Autodesk Inventor part; units mm, degrees
ref_plane "YZ Plane" through (0, 0, 0) normal (1, 0, 0) x (0, 1, 0)
ref_plane "XZ Plane" through (0, 0, 0) normal (0, 1, 0) x (-1, 0, 0)
ref_plane "XY Plane" through (0, 0, 0) normal (0, 0, 1) x (1, 0, 0)
sketch "Szkic1" plane through (0, 0, 0) normal (0, 1, 0) x (-1, 0, 0)
  line L0 (0, 0) -> (0, -35)
  circle A0 centre (0, 0) radius 2
  circle A1 centre (0, -35) radius 2
  line L1 (0, 0) -> (0, -35) construction
  line L2 (-25, 0) -> (-25, -35)
  line L3 (25, -35) -> (25, 0)
  arc A2 (25, 0) -> (-25, 0) centre (0, 0) ccw
  arc A3 (-25, -35) -> (25, -35) centre (0, -35) ccw
  line L4 (-20, -45) -> (20, -45)
  line L5 (20, -45) -> (20, -25)
  line L6 (20, -25) -> (-20, -25)
  line L7 (-20, -25) -> (-20, -45)
  line L8 (-20, -45) -> (20, -25) construction
  line L9 (20, -45) -> (-20, -25) construction
  line L10 (0, -17.5) -> (-25, -17.5) construction
  line L11 (0, -35) -> (0, 0)
  circle A4 centre (0, 0) radius 2
  line L12 (0, -35) -> (0, 0) construction
  line L13 (-20, 10) -> (20, 10)
  line L14 (20, 10) -> (20, -10)
  line L15 (20, -10) -> (-20, -10)
  line L16 (-20, 10) -> (20, -10) construction
  line L17 (20, 10) -> (-20, -10) construction
  line L18 (-20, -10) -> (-20, 10)
  line L19 (0, -17.5) -> (-400, -17.5) construction
  line L20 (0, -17.5) -> (400, -17.5) construction
  line L21 (21.5, 12.5) -> (-21.5, 12.5)
  line L22 (-21.5, 12.5) -> (-21.5, -47.5)
  line L23 (-21.5, -47.5) -> (21.5, -47.5)
  line L24 (21.5, -47.5) -> (21.5, 12.5)
  line L25 (21.5, 12.5) -> (-21.5, -47.5) construction
  line L26 (-21.5, 12.5) -> (21.5, -47.5) construction
  line L27 (21.5, -47.5) -> (28.5, -47.5)
  line L28 (28.5, -47.5) -> (28.5, 12.5)
  line L29 (28.5, 12.5) -> (21.5, 12.5)
  line L30 (21.5, 12.5) -> (21.5, -47.5)
  line L31 (20, 10) -> (20, -10)
  line L32 (20, 0) -> (20, -10)
  circle A5 centre (25, -5) radius 2
  line L33 (20, 0) -> (28.5, 0) construction
  circle A6 centre (25, 5) radius 2
  circle A7 centre (-25, -5) radius 2
  circle A8 centre (-25, 5) radius 2
  line L34 (-21.5, -47.5) -> (-21.5, 12.5)
  line L35 (-21.5, -47.5) -> (-28.5, -47.5)
  line L36 (-28.5, -47.5) -> (-28.5, 12.5)
  line L37 (-28.5, 12.5) -> (-21.5, 12.5)
  circle A9 centre (25, -30) radius 2
  circle A10 centre (25, -40) radius 2
  circle A11 centre (-25, -30) radius 2
  circle A12 centre (-25, -40) radius 2
  point P0 (20, -5)
  dimension "d0" = 35
  dimension "d1" = 4
  dimension "d2" = 4
  dimension "d3" = 50
  dimension "d6" = 40
  dimension "d7" = 20
  dimension "d8" = 400
  dimension "d9" = 180
  dimension "d10" = 43
  dimension "d11" = 60
  dimension "d21" = 7
  dimension "d22" = 60
  dimension "d24" = 4
  dimension "d25" = 5
  dimension "d26" = 5
extrude "Wyciągnięcie proste1" add sketch "Szkic1" against normal blind 5 contours L21 L24 L23 L22
sketch "Szkic2" plane through (-21.5, 0, -47.5) normal (-1, 0, 0) x (0, 0, 1)
  line L0 (22.5, 0) -> (22.5, -5)
  line L1 (37.5, 0) -> (37.5, -5)
  line L2 (22.5, 0) -> (37.5, 0)
  line L3 (30, 0) -> (30, 6)
  line L4 (36, 12) -> (24, 12)
  line L5 (24, 12) -> (24, 0)
  line L6 (24, 0) -> (36, 0)
  line L7 (36, 0) -> (36, 12)
  line L8 (36, 12) -> (24, 0) construction
  line L9 (24, 12) -> (36, 0) construction
  line L10 (34, 10) -> (26, 10)
  line L11 (26, 10) -> (26, 2)
  line L12 (26, 2) -> (34, 2)
  line L13 (34, 2) -> (34, 10)
  line L14 (34, 10) -> (26, 2) construction
  line L15 (26, 10) -> (34, 2) construction
  point P0 (47.5, 0)
  point P1 (36, 0)
  point P2 (24, 0)
  dimension "d12" = 6
  dimension "d13" = 12
  dimension "d14" = 12
  dimension "d15" = 8
  dimension "d16" = 8
extrude "Wyciągnięcie proste2" add sketch "Szkic2" against normal up to surface (43 mm away)
fillet "Zaokrąglenie2" radius 3 2 edges at (0, 12, -11.5) (0, 12, -23.5)
extrude "Wyciągnięcie proste3" add sketch "Szkic1" against normal blind 5 contours A2 A8 L37 L22 L35 A3 A12 L2 A11 A7 | L2 A7 A11 A3 A12 L35 L36 L37 A2 A8 | L29 L28 L27 A3 A10 L3 A9 A5 A2 A6 | A2 A6 L3 A5 A9 A3 A10 L27 L24 L29
sketch "Szkic3" plane through (-21.5, 0, -23.5) normal (-1, 0, 0) x (0, 0, 1)
  line L0 (10, 2) -> (2, 2) construction
  line L1 (2, 10) -> (10, 10) construction
  line L2 (10, 2) -> (2, 10) construction
  line L3 (10, 10) -> (10, 2) construction
  line L4 (2, 2) -> (10, 10) construction
  line L5 (2, 10) -> (10, 10) construction
  line L6 (10, 10) -> (10, 2) construction
  line L7 (10, 2) -> (2, 2) construction
  line L8 (2, 2) -> (2, 10) construction
  line L9 (2, 10) -> (10, 2) construction
  line L10 (10, 10) -> (2, 2) construction
  point P0 (23.5, 0)
  point P1 (6, 6)
sketch "Szkic4" plane through (0, -5, 0) normal (0, -1, 0) x (1, 0, 0)
  line L0 (20, -10) -> (20, 10)
  line L1 (20, 0) -> (20, 0.8)
  line L2 (20, 0) -> (22.1856, 0) construction
  line L3 (20, 0.8) -> (27, 0.8)
  line L4 (27, 0.8) -> (27, 0)
  line L5 (20, 10) -> (20, -10)
  line L6 (20, -0.8) -> (27, -0.8)
  line L7 (27, -0.8) -> (27, 0)
  line L8 (20, 10) -> (-20, 10)
  line L9 (0, 10) -> (0, -45)
  line L10 (-20, -45) -> (20, -45)
  line L11 (28.5, 12.5) -> (28.5, -47.5)
  line L12 (28.5, -17.5) -> (-28.5, -17.5)
  line L13 (-28.5, -47.5) -> (-28.5, 12.5)
  line L14 (-20, -10) -> (-20, 10)
  line L15 (-20, 0) -> (-20, 0.8)
  line L16 (-20, 0) -> (-22.1856, 0) construction
  line L17 (-20, 0.8) -> (-27, 0.8)
  line L18 (-27, 0.8) -> (-27, 0)
  line L19 (-20, -0.8) -> (-27, -0.8)
  line L20 (-27, -0.8) -> (-27, 0)
  line L21 (20, -25) -> (20, -45)
  line L22 (20, -35) -> (20, -35.8)
  line L23 (20, -35) -> (22.1856, -35) construction
  line L24 (20, -35.8) -> (27, -35.8)
  line L25 (20, -34.2) -> (27, -34.2)
  line L26 (20, -45) -> (20, -25)
  line L27 (20, -45) -> (-20, -45)
  line L28 (-20, -35) -> (-20, -35.8)
  line L29 (-20, -35) -> (-22.1856, -35) construction
  line L30 (-20, -34.2) -> (-27, -34.2)
  line L31 (-20, -25) -> (-20, -45)
  line L32 (-20, -35.8) -> (-27, -35.8)
  line L33 (27, -34.2) -> (27, -35.8)
  line L34 (-27, -34.2) -> (-27, -35.8)
  point P0 (0, 0)
  point P1 (0, -35)
  dimension "d29" = 0.8
  dimension "d30" = 7
extrude "Wyciągnięcie proste4" cut sketch "Szkic4" against normal blind 10
sketch "Szkic5" plane through (0, -5, 0) normal (0, -1, 0) x (1, 0, 0)
  line L0 (-20, -35.8) -> (-27, -35.8)
  line L1 (-27, -35.8) -> (-27, -34.2)
  line L2 (-27, -34.2) -> (-20, -34.2)
  line L3 (-20, -34.2) -> (-20, -25)
  line L4 (-20, -25) -> (20, -25)
  line L5 (20, -25) -> (20, -34.2)
  line L6 (20, -34.2) -> (27, -34.2)
  line L7 (27, -34.2) -> (27, -35.8)
  line L8 (27, -35.8) -> (20, -35.8)
  line L9 (20, -35.8) -> (20, -45)
  line L10 (20, -45) -> (-20, -45)
  line L11 (-20, -45) -> (-20, -35.8)
  line L12 (28.5, 12.5) -> (-28.5, 12.5)
  line L13 (-28.5, 12.5) -> (-28.5, -47.5)
  line L14 (-28.5, -47.5) -> (28.5, -47.5)
  line L15 (28.5, -47.5) -> (28.5, 12.5)
  circle A0 centre (-25, -40) radius 2
  circle A1 centre (-25, -30) radius 2
  circle A2 centre (-25, -5) radius 2
  circle A3 centre (-25, 5) radius 2
  circle A4 centre (25, 5) radius 2
  circle A5 centre (25, -5) radius 2
  circle A6 centre (25, -30) radius 2
  circle A7 centre (25, -40) radius 2
  line L16 (-27, 0.8) -> (-20, 0.8)
  line L17 (-20, 0.8) -> (-20, 10)
  line L18 (-20, 10) -> (20, 10)
  line L19 (20, 10) -> (20, 0.8)
  line L20 (20, 0.8) -> (27, 0.8)
  line L21 (27, 0.8) -> (27, -0.8)
  line L22 (27, -0.8) -> (20, -0.8)
  line L23 (20, -0.8) -> (20, -10)
  line L24 (20, -10) -> (-20, -10)
  line L25 (-20, -10) -> (-20, -0.8)
  line L26 (-20, -0.8) -> (-27, -0.8)
  line L27 (-27, -0.8) -> (-27, 0.8)
  point P0 (0, 0)
properties part number "base"
Part model, mm, in its own coordinate system. A direction names the side the tool comes from. Coordinates: 2 decimals unless noted, no trailing zeros. Order: outer loops, then holes, each group sorted by start corner. A loop starts at its lowest first (then second) coordinate and runs counter-clockwise, first axis right, second up. Notation, with made-up numbers: (-30.75, -15) - (13.25, -15) arc R6 cw to (13.25, -7) - close; hole circle Ø11 at (4.5, 16.5). An arc over 180 degrees is marked (long way). Return JSON: item names as keys, results as strings. Group by question number.
Item 1: Which spindle directions (+Z, -Z, +X, -X, +Y, -Y) get a long thin tool onto all of the face, cutting with end or side? Do faces 5 (the face through (23, -3, -34.2)), 6 (the face through (0, -2, 12.5)). Say none if no direction does.
Item 2: Cut at D-D (z = -40). List the corners of the cut face in (x, y).
Item 3: Pull direction X, two halves, no side cores. Call faces 1 (the face through (-23, -3, 0.8)), 2 (the face through (-23, -2, 5)), 3 (the face through (-28.5, -2, -18)), 4 (the face through (0, 4, -11.5)): pulls with the +X half, pulls with the -X half, needs draft (parallel to the pull), parting line crosses it, or undercut.
Item 4: Pin check, flat tips, straight feed: pin 1 (4.5 mm diameter, centred on x = 25, z = -40, fed in from +Y); pin 2 (2.5 mm diameter, centred on x = 9.5, y = 6.5, fed in from -Z). Stop position of each tip, or through.
Item 5: Cut at A-A (x = 9.5). List the corners of the cut face in (y, z).
Item 6: Cut at C-C (x = -25). List the corners of the cut face in (y, z).
Item 7: Drill centre lines: probe 1 along Z at (x, y) = (18, -2.75); probe 2 along X at (y, z) = (-1.3, 5); probe 3 along Y at (x, z) = (6.5, -18). Where is each one in solid material? Low to high. Write a range as from..to.
Item 8: Cut at B-B (z = -16). List the corners of the cut face in (x, y), plus the area to 3 significant figures.
Check values:
{
 "1": {"face 5": "+Y, -Y", "face 6": "+Z, +X, -X, +Y, -Y"},
 "2": {"outline": "(-28.5, -5) - (-27, -5) - (-27, 0) - (-28.5, 0) - close; (-23, -5) - (-20, -5) - (-20, 0) - (-23, 0) - close; (20, -5) - (23, -5) - (23, 0) - (20, 0) - close; (27, -5) - (28.5, -5) - (28.5, 0) - (27, 0) - close"},
 "3": {"face 1": "undercut", "face 2": "undercut", "face 3": "pulls with the -X half", "face 4": "needs draft"},
 "4": {"pin 1": "stops at y = 0", "pin 2": "stops at z = -23.5"},
 "5": {"outline": "(-5, -47.5) - (0, -47.5) - (0, -45) - (-5, -45) - close; (-5, -25) - (0, -25) - (0, -23.5) - (9, -23.5) arc R3 ccw to (12, -20.5) - (12, -14.5) arc R3 ccw to (9, -11.5) - (0, -11.5) - (0, -10) - (-5, -10) - close; (-5, 10) - (0, 10) - (0, 12.5) - (-5, 12.5) - close; hole (2, -21.5) - (10, -21.5) - (10, -13.5) - (2, -13.5) - close"},
 "6": {"outline": "(-5, -47.5) - (0, -47.5) - (0, -42) - (-5, -42) - close; (-5, -38) - (0, -38) - (0, -35.8) - (-5, -35.8) - close; (-5, -34.2) - (0, -34.2) - (0, -32) - (-5, -32) - close; (-5, -28) - (0, -28) - (0, -7) - (-5, -7) - close; (-5, -3) - (0, -3) - (0, -0.8) - (-5, -0.8) - close; (-5, 0.8) - (0, 0.8) - (0, 3) - (-5, 3) - close; (-5, 7) - (0, 7) - (0, 12.5) - (-5, 12.5) - close"},
 "7": {"probe 1": "z = -47.5..-45, -25..-10, 10..12.5", "probe 2": "x = -28.5..-27, -23..-20, 20..23, 27..28.5", "probe 3": "y = -5..2, 10..12"},
 "8": {"outline": "(-28.5, -5) - (28.5, -5) - (28.5, 0) - (21.5, 0) - (21.5, 2) - (-21.5, 2) - (-21.5, 0) - (-28.5, 0) - close; (-21.5, 10) - (21.5, 10) - (21.5, 12) - (-21.5, 12) - close", "area": "457 mm2"}
}
